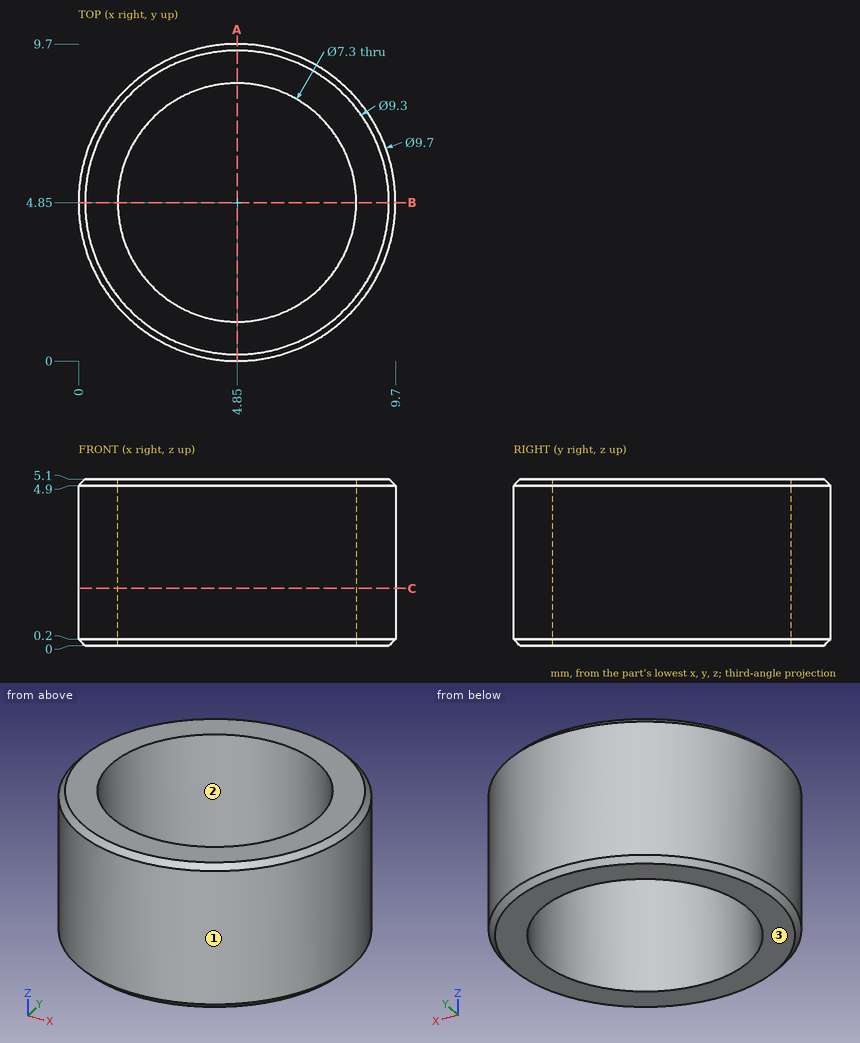
Could you check a few things on this drawing? It's one solid part, dimensions in mm from its lowest x, y, z. Give positions to 0.01 mm unless a question says otherwise; leave off trailing zeros. Order: outer loops, then holes, each group sorted by start corner. A loop starts at its lowest first (then second) coordinate and runs counter-clockwise, first axis right, second up. Notation, with made-up numbers: (68.25, -21) - (114.25, -21) arc R32 cw to (114.25, 6) - close; hole circle Ø9 at (-35, 75). An arc over 180 degrees is marked (long way). One line per question, with ' | ' between items. Start each with the question number.
Item 1: Thinking about a two-plate mould opening in X: for the marked faces 1, 2 and 3, which applies, pulls with the +X half, pulls with the -X half, needs draft (parallel to the pull), parting line crosses it, or undercut?
Item 2: I'm going to push flat-ended pins straight in: pin 1 Ø1 at (y, z) = (6.5, 3) entering from +X; pin 2 Ø2 at (x, z) = (3, 3.5) entering from +Y; pin 3 Ø3 at (x, y) = (3, 6.5) entering from +Z; pin 4 Ø3 at (y, z) = (6.5, 1.5) entering from +X. Where does each tip first touch, or does it pass through?
Item 3: I want a section at C-C on z = 1.75. Write out the boundary of the cut face in (x, y), then the cut area to 3 significant figures.
Item 4: I need wall thicknesses on probe 1 along Y at (x, z) = (4.85, 3.5); probe 2 along X at (y, z) = (3, 0.4); probe 3 along X at (y, z) = (4.5, 2.65). Which ranges of each line are inside material? Lowest first, please. Write a range as [from, to].
Item 5: I want a section at A-A on x = 4.85. Write out the boundary of the cut face in (y, z), then the cut area to 3 significant figures.
Verdict:
1) face 1: parting line crosses it | face 2: undercut | face 3: needs draft
2) pin 1: x = 9.56 | pin 2: y = 9.62 | pin 3: z = 5.1 | pin 4: x = 9.7
3) outline: circle Ø9.7 at (4.85, 4.85); hole circle Ø7.3 at (4.85, 4.85) | area: 32.0 mm^2
4) probe 1: [0, 1.2], [8.5, 9.7] | probe 2: [0.37, 1.7], [8, 9.33] | probe 3: [0.01, 1.22], [8.48, 9.69]
5) outline: (0, 0.2) - (0.2, 0) - (1.2, 0) - (1.2, 5.1) - (0.2, 5.1) - (0, 4.9) - close; (8.5, 0) - (9.5, 0) - (9.7, 0.2) - (9.7, 4.9) - (9.5, 5.1) - (8.5, 5.1) - close | area: 12.2 mm^2
